Source: three-view drawing plus pictorial views. Frame: mm from the lowest corner of the part. A direction names the side the tool comes from. Give positions to 0.01 mm unless a question says otherwise; leave off trailing zeros. Order: outer loops, then holes, each group sorted by start corner. A loop starts at its lowest first (then second) coordinate and runs counter-clockwise, first axis right, second up. Notation, with made-up numbers: (25.25, 75) - (74.25, 75) arc R35 ccw to (74.25, 108) - close; hole circle Ø9 at (22.25, 49.5). An arc over 180 degrees is marked (long way). Answer in a Markdown table with one row per item. Add a question column.
1. Section query B-B on y = 2.4. Return loops of the section in (x, z), and give its area (3 significant figures).
2. Contact query for flat-ended pins moving along their axis: pin 1 (2 mm diameter, centred on x = 13, y = 3.5, fed in from -Z); pin 2 (1.6 mm diameter, centred on y = 3, z = 9.5, fed in from +X). Output: stop coordinate, or through.
3. Section query D-D on x = 17.25. Return loops of the section in (y, z).
4. Section query A-A on z = 12.5. Return loops of the section in (x, y).
5. Access query for the marked faces 1, 2, 3 and 4. Directions: +Z, -Z, +X, -X, +Y, -Y. A direction counts if a zero-diameter tool reaches every point of the face in a straight line with its end or side. Return the directions, or none.
6. Ray query, line 1 (Z direction, x = 7.25, y = 1.9); line 2 (X direction, y = 3.6, z = 11.5). Return the intervals inside material, ascending. Write a range as [from, to].
7. Section query C-C on x = 14. Return loops of the section in (y, z), and give its area (3 significant figures).
8. Mould query, pull axis Z, two halves, no side actions, for the marked faces 5, 6 and 7. Classes: released by +Z, released by -Z, zero draft, split by the parting line, or undercut.
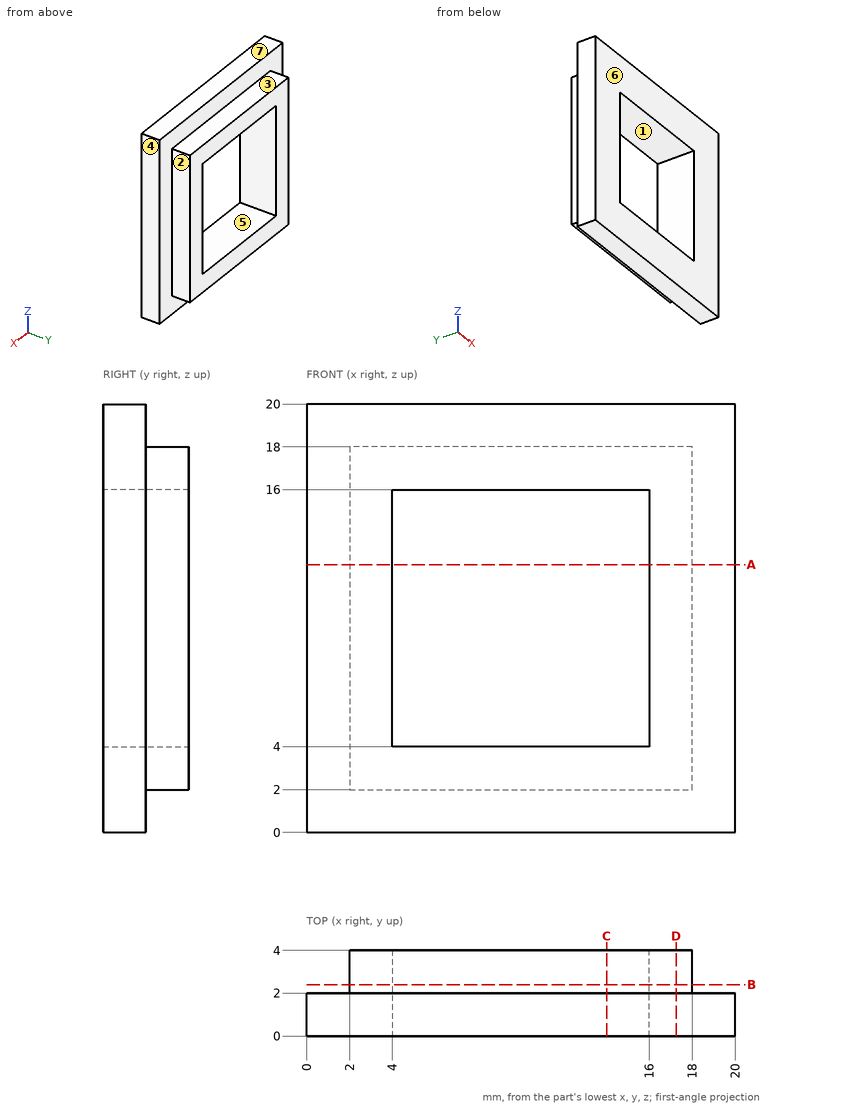
Answer:
| question | item | result |
|---|---|---|
| 1 | outline | (2, 2) - (18, 2) - (18, 18) - (2, 18) - close; hole (4, 4) - (16, 4) - (16, 16) - (4, 16) - close |
| 1 | area | 112 mm² |
| 2 | pin 1 | stops at z = 2 |
| 2 | pin 2 | stops at x = 18 |
| 3 | outline | (0, 0) - (2, 0) - (2, 2) - (4, 2) - (4, 18) - (2, 18) - (2, 20) - (0, 20) - close |
| 4 | outline | (0, 0) - (4, 0) - (4, 4) - (2, 4) - (2, 2) - (0, 2) - close; (16, 0) - (20, 0) - (20, 2) - (18, 2) - (18, 4) - (16, 4) - close |
| 5 | face 1 | +Y, -Y |
| 5 | face 2 | +Z, -Z, +X, +Y |
| 5 | face 3 | +Z, +X, -X, +Y |
| 5 | face 4 | +Z, -Z, +X, +Y, -Y |
| 6 | line 1 | z = [0, 4], [16, 20] |
| 6 | line 2 | x = [2, 4], [16, 18] |
| 7 | outline | (0, 0) - (2, 0) - (2, 2) - (4, 2) - (4, 4) - (0, 4) - close; (0, 16) - (4, 16) - (4, 18) - (2, 18) - (2, 20) - (0, 20) - close |
| 7 | area | 24.0 mm² |
| 8 | face 5 | undercut |
| 8 | face 6 | zero draft |
| 8 | face 7 | released by +Z |
